Autodesk Inventor part; units mm, degrees
ref_plane "YZ Plane" through (0, 0, 0) normal (1, 0, 0) x (0, 1, 0)
ref_plane "XZ Plane" through (0, 0, 0) normal (0, 1, 0) x (-1, 0, 0)
ref_plane "XY Plane" through (0, 0, 0) normal (0, 0, 1) x (1, 0, 0)
sketch "Sketch1" plane through (0, 0, 0) normal (0, 1, 0) x (-1, 0, 0)
  circle A0 centre (0, 35.3) radius 1.55
  circle A1 centre (18, -36) radius 1.55
  circle A2 centre (-18, -36) radius 1.55
  circle A3 centre (0, 35.3) radius 5
  circle A4 centre (18, -36) radius 5
  circle A5 centre (-18, -36) radius 5
  point P0 (0, 0)
  dimension "d0" = 35.3
  dimension "d1" = 36
  dimension "d2" = 3.1
  dimension "d3" = 10
  dimension "d4" = 36
  dimension "d5" = 18
extrude "Extrusion1" add sketch "Sketch1" along normal blind 15
sketch "Sketch2" plane through (0, 0, 35.3) normal (0, -1, 0) x (1, 0, 0)
  circle A0 centre (0, 0) radius 5
  circle A1 centre (0, 0) radius 1.55
  circle A2 centre (-18, -71.3) radius 1.55
  circle A3 centre (-18, -71.3) radius 5
  circle A4 centre (18, -71.3) radius 1.55
  circle A5 centre (18, -71.3) radius 5
  line L0 (-22.8479, -70.0761) -> (-4.8479, 1.2239)
  line L1 (22.8479, -70.0761) -> (4.8479, 1.2239)
  line L2 (-18, -76.3) -> (18, -76.3)
  circle A6 centre (0, -35.3) radius 2.1
  dimension "d8" = 4.2
extrude "Extrusion2" add sketch "Sketch2" along normal blind 3
sketch "Sketch3" plane through (0, 0, 35.3) normal (0, 1, 0) x (1, 0, 0)
  circle A0 centre (-30, 5.3) radius 16
  circle A1 centre (0, 35.3) radius 29.9 construction
  line L0 (0, 35.3) -> (-30, 5.3) construction
  line L1 (0, 35.3) -> (-30, 35.3) construction
  circle A2 centre (-30, 5.3) radius 2.1 construction
  line L2 (-28, 9.3) -> (-32, 9.3)
  line L3 (-32, 9.3) -> (-30, 19.3)
  line L4 (-30, 19.3) -> (-28, 9.3)
  line L5 (-27.9, 5.3) -> (-32.1, 5.3) construction
  line L6 (-30, 3.2) -> (-30, 7.4) construction
  line L7 (-30, 5.3) -> (-30, 35.3) construction
  line L8 (-26, 3.3) -> (-26, 7.3)
  line L9 (-26, 7.3) -> (-16, 5.3)
  line L10 (-16, 5.3) -> (-26, 3.3)
  line L11 (-24.3431, 8.1284) -> (-27.1716, 10.9569)
  line L12 (-27.1716, 10.9569) -> (-21.5147, 13.7853)
  line L13 (-24.3431, 8.1284) -> (-21.5147, 13.7853)
  circle A3 centre (-30, 5.3) radius 2.1
  line L14 (-24.3431, 2.4716) -> (-27.1716, -0.3569)
  line L15 (-27.1716, -0.3569) -> (-21.5147, -3.1853)
  line L16 (-24.3431, 2.4716) -> (-21.5147, -3.1853)
  line L17 (-35.6569, 8.1284) -> (-32.8284, 10.9569)
  line L18 (-32.8284, 10.9569) -> (-38.4853, 13.7853)
  line L19 (-35.6569, 8.1284) -> (-38.4853, 13.7853)
  line L20 (-35.6569, 2.4716) -> (-38.4853, -3.1853)
  line L21 (-32.8284, -0.3569) -> (-38.4853, -3.1853)
  line L22 (-35.6569, 2.4716) -> (-32.8284, -0.3569)
  line L23 (-34, 3.3) -> (-34, 7.3)
  line L24 (-34, 7.3) -> (-44, 5.3)
  line L25 (-44, 5.3) -> (-34, 3.3)
  line L26 (-28, 1.3) -> (-32, 1.3)
  line L27 (-32, 1.3) -> (-30, -8.7)
  line L28 (-30, -8.7) -> (-28, 1.3)
  circle A4 centre (0, 0) radius 5
  line L29 (-4.8479, -1.2239) -> (-22.8479, 70.0761)
  line L30 (-13.8479, 34.4261) -> (-27.2178, 21.0562)
  line L31 (-8.1467, 11.8431) -> (-14.0143, 5.9755)
  circle A5 centre (0, 35.3) radius 2.1 construction
  point P0 (-25.7574, 9.5426)
  dimension "d41" = 59.8
  dimension "d49" = 30
  dimension "d50" = 45
  dimension "d51" = 32
  dimension "d52" = 4.2
  dimension "d53" = 4
  dimension "d54" = 10
  dimension "d55" = 4
  dimension "d56" = 4
  dimension "d57" = 4
  dimension "d58" = 6
  dimension "d59" = 6
  dimension "d70" = 20
  dimension "d71" = 45
extrude "Extrusion3" add sketch "Sketch3" against normal blind 3 contours A0 | A0 L30 L29 L31
mirror "Mirror1" about plane through (0, 0, 0) normal (1, 0, 0) of "Extrusion3"
properties part number "BASE_LIDAR" material "ABS Plastic"
Model file for the job. Use its own axes, mm. A direction names the side the tool comes from. Coordinates: 2 decimals unless noted, no trailing zeros. Order: outer loops, then holes, each group sorted by start corner. A loop starts at its lowest first (then second) coordinate and runs counter-clockwise, first axis right, second up. Notation, with made-up numbers: M 8,-22.75 L 26,-22.75 A13 cw 26,-3.75 Z; hole C 76.5,72 d2. An arc over 180 degrees is marked long. Answer as CSV lines item,"result".
(1) Pull direction X, two halves, no side cores. Call faces 1 (the flat face through (-34.262, -1.479, 34.223)), 2 (the flat face through (-18.41, -1.48, -17.2)), 3 (the flat face through (-18, 15, -38)): +X half, -X half, draft (parallel to the pull), parting line (faces both ways), or undercut.
Geometry says:
face 1,"undercut"
face 2,"-X half"
face 3,"draft"
(2) Flat gauge pins, fed straight in: pin 1 (12 mm diameter, centred on x = 26, z = 34.5, fed in from +Y); pin 2 (1.5 mm diameter, centred on x = -18.5, y = 10.5, fed in from +Z); pin 3 (3.5 mm diameter, centred on y = -2, z = 29, fed in from +X); pin 4 (1 mm diameter, centred on y = 12, z = 32.5, fed in from +X). Where does each tip first touch, or does it go through?
Geometry says:
pin 1,"stops at y = 0"
pin 2,"stops at z = -31"
pin 3,"stops at x = 46"
pin 4,"stops at x = 4.44"
(3) 3-axis set-ups, long thin cutter, end or side, ignore diameter. For faces 4 (the flat face through (18, 15, -38)), 5 (the flat face through (-25.738, -1.479, 34.223)): which of +Z, -Z, +X, -X, +Y, -Y reach the whole face in a straight line?
Geometry says:
face 4,"+Z, -Z, +X, -X, +Y"
face 5,"+Y, -Y"
(4) Band-saw the part on A-A, the plane y = 2. List the corners of the cut face in (x, z), then the cut area to 3 significant figures.
Geometry says:
outline,"C -18,-36 d10; C 0,35.3 d10; C 18,-36 d10; hole C -18,-36 d3.1; hole C 0,35.3 d3.1; hole C 18,-36 d3.1"
area,"213 mm2"
(5) Band-saw the part on C-C, the plane x = 0. List the corners of the cut face in (y, z), then the cut area to 4 significant figures.
Geometry says:
outline,"M -3,-41 L 0,-41 L 0,-2.1 L -3,-2.1 Z; M -3,2.1 L 0,2.1 L 0,30.3 L 15,30.3 L 15,33.75 L -3,33.75 Z; M -3,36.85 L 15,36.85 L 15,40.3 L -3,40.3 Z"
area,"325.5 mm2"
(6) Band-saw the part on D-D, the plane z = -17.5. List the corners of the cut face in (x, y).
Geometry says:
outline,"M -18.49,-3 L 18.49,-3 L 18.49,0 L -18.49,0 Z"
(7) Band-saw the part on B-B, the plane x = -37. List the corners of the cut face in (y, z).
Geometry says:
outline,"M -3,15.61 L 0,15.61 L 0,22.26 L -3,22.26 Z; M -3,24.49 L 0,24.49 L 0,28.6 L -3,28.6 Z; M -3,31.4 L 0,31.4 L 0,35.51 L -3,35.51 Z; M -3,37.74 L 0,37.74 L 0,44.39 L -3,44.39 Z"
(8) Wall check: line 1 along Z through (x, y) = (0, -0.85); line 2 along X through (y, z) = (-2.35, -36); line 3 along Z through (x, y) = (0, 12). Give the ranges that are in metal, low to high.
Geometry says:
line 1,"z = -41 to -2.1, 2.1 to 33.75, 36.85 to 40.3"
line 2,"x = -23 to -19.55, -16.45 to 16.45, 19.55 to 23"
line 3,"z = 30.3 to 33.75, 36.85 to 40.3"
